Model file for the job. Use its own axes, mm. A direction names the side the tool comes from. Round coordinates to 2 decimals unless told otherwise and drop trailing zeros. Order: outer loops, then holes, each group sorted by start corner. A loop starts at its lowest first (then second) coordinate and runs counter-clockwise, first axis right, second up. Notation, with made-up numbers: (73.5, 18.25) - (132.5, 18.25) arc R11 cw to (132.5, 28.25) - close; hole circle Ø1 at (-16, 6.5). An arc over 180 degrees is marked (long way). Put each result on its own line as item: value. Start each with the question number.
Item 1: Saw through at B-B on y = 520. List the corners of the cut face in (x, z), plus the area to 3 significant figures.
Item 2: Saw through at D-D on y = 288. List the corners of the cut face in (x, z), plus the area to 3 significant figures.
Item 3: Mould opens along Z. For faces 6 (the face through (267.605, 501.403, 184.13)), 7 (the face through (-4, 720, -4)), 8 (the face through (218, 629, -260)), 9 (the face through (264, 385, 275)) say: pulls with the +Z half, pulls with the -Z half, needs draft (parallel to the pull), parting line crosses it, or undercut.
Item 4: Saw through at A-A on z = 214.5. List the corners of the cut face in (x, y).
Item 5: Which spindle directions (+Z, -Z, +X, -X, +Y, -Y) get a long thin tool onto all of the face, cutting with end or side? Do faces 1 (the face through (275, 275, 4)), 2 (the face through (-267.605, 501.403, -184.13)), 3 (the face through (-275, 355, 4)), 4 (the face through (-260, 355, 11)), 5 (the face through (209, 629, 260)). Say none if no direction does.
Item 6: Probe probe 1 along Y at (x, z) = (263, 180); probe 2 along Y at (x, z) = (191, 135.5); probe 3 along X at (y, z) = (349, -95). List the from-to ranges inside material, lowest first.
Item 7: Saw through at C-C on x = 84. List the corners of the cut face in (y, z).
```python
from build123d import *

# Parameters (mm, degrees)
CROQUIS1_W              = 550
CROQUIS1_H              = 550
SALIENTE_EXTRUIR1_DEPTH = 720
VACIADO1_T              = -15
SALIENTE_EXTRUIR2_DEPTH = 535
CROQUIS3_W              = 505
CROQUIS3_H              = 150
CORTAR_EXTRUIR1_DEPTH   = 115
CROQUIS4_W              = 15
CROQUIS4_H              = 150
SALIENTE_EXTRUIR3_DEPTH = 100
CROQUIS5_R              = 19.05
CORTAR_EXTRUIR2_DEPTH   = 30
CROQUIS6_R              = 19.05
CORTAR_EXTRUIR3_DEPTH   = 30


with BuildPart() as part:
    # Croquis1 → Saliente-Extruir1 (new body)
    with BuildSketch(Plane(origin=(0, 0, 0), x_dir=(1, 0, 0), z_dir=(0, 1, 0))):
        Rectangle(CROQUIS1_W, CROQUIS1_H)
    extrude(amount=SALIENTE_EXTRUIR1_DEPTH)

    # Vaciado1
    vaciado1_openings = [part.faces().sort_by_distance(p)[0] for p in [
        (0, 360, 275),
    ]]
    offset(amount=VACIADO1_T, openings=vaciado1_openings, kind=Kind.INTERSECTION)

    # Croquis2 → Saliente-Extruir2 (add)
    with BuildSketch(Plane.XY.offset(275)):
        Polygon((160, 705), (160, 555), (260, 555), (260, 540), (145, 540), (145, 705), align=None)
    extrude(amount=-SALIENTE_EXTRUIR2_DEPTH)

    # Croquis3 → Cortar-Extruir1 (cut)
    with BuildSketch(Plane(origin=(275, 0, 0), x_dir=(0, 0, -1), z_dir=(1, 0, 0))):
        with Locations((7.5, 630)):
            Rectangle(CROQUIS3_W, CROQUIS3_H)
    extrude(amount=-CORTAR_EXTRUIR1_DEPTH, mode=Mode.SUBTRACT)

    # Croquis4 → Saliente-Extruir3 (add)
    with BuildSketch(Plane(origin=(160, 0, 0), x_dir=(0, 0, -1), z_dir=(1, 0, 0))):
        with Locations((-267.5, 630)):
            Rectangle(CROQUIS4_W, CROQUIS4_H)
    extrude(amount=SALIENTE_EXTRUIR3_DEPTH)

    # Croquis5 → Cortar-Extruir2 (cut)
    with BuildSketch(Plane.ZY.offset(275)):
        with Locations((-180, 520)):
            Circle(CROQUIS5_R)
    extrude(amount=-CORTAR_EXTRUIR2_DEPTH, mode=Mode.SUBTRACT)

    # Croquis6 → Cortar-Extruir3 (cut)
    with BuildSketch(Plane(origin=(275, 0, 0), x_dir=(0, 0, -1), z_dir=(1, 0, 0))):
        with Locations((-180, 520)):
            Circle(CROQUIS6_R)
    extrude(amount=-CORTAR_EXTRUIR3_DEPTH, mode=Mode.SUBTRACT)


solid = part.part
```
Results found:
1. outline: (-275, -275) - (275, -275) - (275, 160.95) - (260, 160.95) - (260, -260) - (-260, -260) - (-260, -199.05) - (-275, -199.05) - close; (-275, -160.95) - (-260, -160.95) - (-260, 275) - (-275, 275) - close; (260, 199.05) - (275, 199.05) - (275, 275) - (260, 275) - close
1. area: 23,200 mm²
2. outline: (-275, -275) - (275, -275) - (275, 275) - (260, 275) - (260, -260) - (-260, -260) - (-260, 275) - (-275, 275) - close
2. area: 24,300 mm²
3. face 6: undercut
3. face 7: needs draft
3. face 8: undercut
3. face 9: pulls with the +Z half
4. outline: (-275, 0) - (275, 0) - (275, 555) - (160, 555) - (160, 705) - (275, 705) - (275, 720) - (-275, 720) - close; hole (-260, 15) - (260, 15) - (260, 540) - (145, 540) - (145, 705) - (-260, 705) - close
5. face 1: +Z, -Z, +X, +Y, -Y
5. face 2: -X
5. face 3: +Z, -Z, -X, +Y, -Y
5. face 4: +Z
5. face 5: none
6. probe 1: y = 0 to 500.95, 539.05 to 555, 705 to 720
6. probe 2: y = 0 to 15, 540 to 555, 705 to 720
6. probe 3: x = -275 to -260, 260 to 275
7. outline: (0, -275) - (720, -275) - (720, 275) - (705, 275) - (705, -260) - (15, -260) - (15, 275) - (0, 275) - close
